Read the model definition and answer for the solid it produces. Units are mm, in the model's axes. A direction names the side the tool comes from. Give positions to 0.01 mm unless a question says otherwise; leave off trailing zeros. Write each loop counter-clockwise with the first axis right and the second up, starting at its lowest first coordinate (ties: lowest second). Pieces come first, ordered by that corner, then holes. Notation, with made-up numbers: (-24.5, 57.5) -> (17.5, 57.5) arc R13 ccw to (17.5, 65.5) -> close; hole circle Ø4 at (51.5, 30.25). An arc over 180 degrees is marked (long way). Use a Markdown table: item, result.
Autodesk Inventor part; units mm, degrees
ref_plane "YZ Plane" through (0, 0, 0) normal (1, 0, 0) x (0, 1, 0)
ref_plane "XZ Plane" through (0, 0, 0) normal (0, 1, 0) x (-1, 0, 0)
ref_plane "XY Plane" through (0, 0, 0) normal (0, 0, 1) x (1, 0, 0)
sketch "Sketch1" plane through (0, 0, 0) normal (0, 0, 1) x (1, 0, 0)
  line L0 (0, 0) -> (25.4, 0)
  line L1 (25.4, 0) -> (25.4, 25.4)
  line L2 (25.4, 25.4) -> (0, 25.4)
  line L3 (0, 25.4) -> (0, 0)
  line L4 (3.175, 3.175) -> (22.225, 3.175)
  line L5 (22.225, 3.175) -> (22.225, 22.225)
  line L6 (22.225, 22.225) -> (3.175, 22.225)
  line L7 (3.175, 22.225) -> (3.175, 3.175)
  dimension "d0" = 25.4
  dimension "d1" = 25.4
  dimension "d2" = 19.05
  dimension "d3" = 19.05
  dimension "d4" = 3.175
  dimension "d5" = 3.175
extrude "Extrusion1" add sketch "Sketch1" along normal blind 307.975
sketch "Sketch2" plane through (0, 25.4, 0) normal (0, 1, 0) x (1, 0, 0)
  line L0 (25.4, -307.975) -> (0, -307.975)
  line L1 (25.4, 0) -> (25.4, -307.975)
  point P0 (12.7, -295.275)
  point P1 (12.7, -269.875)
  point P2 (12.7, -117.475)
  point P3 (12.7, -92.075)
  dimension "d8" = 12.7
  dimension "d9" = 12.7
  dimension "d11" = 12.7
  dimension "d16" = 12.7
  dimension "d17" = 12.7
  dimension "d34" = 152.4
  dimension "d35" = 25.4
  dimension "d36" = 25.4
hole "Hole1" at (12.7, 25.4, 295.275) at (12.7, 25.4, 269.875) at (12.7, 25.4, 117.475) at (12.7, 25.4, 92.075) direction (0, -1, 0) diameter 6.35 end through all
sketch "Sketch3" plane through (25.4, 0, 0) normal (1, 0, 0) x (0, 0, -1)
  line L0 (0, 0) -> (0, 25.4)
  line L1 (0, 0) -> (-307.975, 0)
  point P0 (-38.1, 12.7)
  dimension "d25" = 38.1
  dimension "d26" = 12.7
hole "Hole2" at (25.4, 12.7, 38.1) direction (-1, 0, 0) diameter 9.525 end through all
sketch "Sketch4" plane through (0, 0, 0) normal (-1, 0, 0) x (0, 0, 1)
  circle A0 centre (38.1, 12.7) radius 4.7625
  circle A1 centre (38.1, 12.7) radius 6.35
  dimension "d37" = 12.7
extrude "Extrusion2" cut sketch "Sketch4" against normal blind 12.7
properties part number "1x1 lengthwise" material "Aluminum 6061"
Item 1: A tool of negligible diameter and unlimited length cuts with its end or side. For faces 1 (the face through (11.746, 23.79, 272.903)), 2 (the face through (13, 3.175, 152)), from which of +Z, -Z, +X, -X, +Y, -Y can it reach the whole face along a straight path? Write none if from no direction.
Return value:
| item | result |
|---|---|
| face 1 | +Y, -Y |
| face 2 | +Z, -Z |
Item 2: Straight lines are drawn through the part: line 1 along Z through (x, y) = (12.7, 2.55) (3 decimals); line 2 along X through (y, z) = (8, 125.5) (3 decimals). For each, find the intervals that lie inside material, in ascending order. Write a range as [from, to].
Return value:
| item | result |
|---|---|
| line 1 | [0, 88.9], [95.25, 114.3], [120.65, 266.7], [273.05, 292.1], [298.45, 307.975] |
| line 2 | [0, 3.175], [22.225, 25.4] |
Item 3: A cutting plane is placed at B-B (y = 12.7). Count the separate pieces of the cut face and the enclosed holes in it, then the cut area to 3 significant figures.
Return value:
| item | result |
|---|---|
| separate pieces | 4 |
| enclosed holes | 0 |
| area | 1,890 mm^2 |
Item 4: A cutting plane is placed at C-C (z = 256.5). Give the vertices of the cut face in (x, y) (3 decimals), then the cut area to 3 significant figures.
Return value:
| item | result |
|---|---|
| outline | (0, 0) -> (25.4, 0) -> (25.4, 25.4) -> (0, 25.4) -> close; hole (3.175, 3.175) -> (22.225, 3.175) -> (22.225, 22.225) -> (3.175, 22.225) -> close |
| area | 282 mm^2 |
Item 5: For a pull along Z with two mould halves and no side action, classify faces 3 (the face through (0, 13, 152)), 4 (the face through (1.565, 12.979, 31.756)), 5 (the face through (12.6, 23.8, 114.3)), 6 (the face through (24, 13, 307.975)) as +Z half, -Z half, draft (parallel to the pull), parting line (faces both ways), or undercut.
Return value:
| item | result |
|---|---|
| face 3 | draft |
| face 4 | undercut |
| face 5 | undercut |
| face 6 | +Z half |
